```python
from build123d import *

# Parameters (mm, degrees)
BOSS_EXTRUDE1_DEPTH = 3.95
SKETCH2_R           = 3.575
CUT_EXTRUDE1_DEPTH  = 3.95
BOSS_EXTRUDE2_DEPTH = 1.64
SKETCH4_R           = 3.25
CUT_EXTRUDE2_DEPTH  = 63.643819328
CAVITY1_OUTLINE_R   = 3.25
CAVITY1_DEPTH       = 5.59
CAVITY1_START       = 3.19
CAVITY1_2_DEPTH     = 2.4
CUT_EXTRUDE4_DEPTH  = 63.643819328
BOSS_EXTRUDE3_START = -5.59
BOSS_EXTRUDE3_DEPTH = 5.59
BOSS_EXTRUDE4_DEPTH = 5.59
BOSS_EXTRUDE5_DEPTH = 5.59
CUT_EXTRUDE5_DEPTH  = 2.4
SKETCH7_R           = 1
CUT_EXTRUDE6_DEPTH  = 5.59


# Read off the part's stored shape, not the designer's step: Cavity1
with BuildPart() as part:
    # Sketch1 → Boss-Extrude1 (new body)
    with BuildSketch(Plane(origin=(0, 0, 0), x_dir=(1, 0, 0), z_dir=(0, 1, 0))):
        with BuildLine():
            Line((0, 7), (55, 7))
            ThreePointArc((55, 7), (62, 0), (55, -7))
            Line((55, -7), (0, -7))
            ThreePointArc((0, -7), (-7, 0), (0, 7))
        make_face()
    extrude(amount=BOSS_EXTRUDE1_DEPTH)

    # Sketch2 → Cut-Extrude1 (cut)
    with BuildSketch(Plane.XZ):
        with Locations(Location((0, 0, 0), (0, 0, 270))):
            Circle(SKETCH2_R)
    extrude(amount=-CUT_EXTRUDE1_DEPTH, mode=Mode.SUBTRACT)

    # Sketch3 → Boss-Extrude2 (add)
    with BuildSketch(Plane(origin=(0, 3.95, 0), x_dir=(1, 0, 0), z_dir=(0, 1, 0))):
        with BuildLine():
            Line((0, -7), (55, -7))
            ThreePointArc((55, -7), (62, 0), (55, 7))
            Line((55, 7), (0, 7))
            ThreePointArc((0, 7), (-7, 0), (0, -7))
        make_face()
        with BuildLine():
            Line((13.979308982, 2.569996388), (1.997926282, 3.167540934))
            ThreePointArc((1.997926282, 3.167540934), (-3.745, 0), (1.997926282, -3.167540934))
            Line((1.997926282, -3.167540934), (13.979308982, -2.569996388))
            ThreePointArc((13.979308982, -2.569996388), (16.545, 0), (13.979308982, 2.569996388))
        make_face(mode=Mode.SUBTRACT)
    extrude(amount=BOSS_EXTRUDE2_DEPTH)

    # Sketch4 → Cut-Extrude2 (cut, through all)
    with BuildSketch(Plane(origin=(0, 5.59, 0), x_dir=(1, 0, 0), z_dir=(0, 1, 0))):
        with Locations(Location((55, 0, 0), (0, 0, 270))):
            Circle(SKETCH4_R)
    extrude(amount=-CUT_EXTRUDE2_DEPTH, mode=Mode.SUBTRACT)

    # Cavity1 outline → Cavity1 (cut)
    with BuildSketch(Plane(origin=(0, 0, 0), x_dir=(1, 0, 0), z_dir=(0, 1, 0))):
        with BuildLine():
            Line((58.605551275, 6), (38, 6))
            Line((38, 6), (38, -6))
            Line((38, -6), (58.605551275, -6))
            ThreePointArc((58.605551275, -6), (59.949747468, -4.949747468), (61, -3.605551275))
            Line((61, -3.605551275), (61, 3.605551275))
            ThreePointArc((61, 3.605551275), (59.949747468, 4.949747468), (58.605551275, 6))
        make_face()
        with Locations((55, 0)):
            Circle(CAVITY1_OUTLINE_R, mode=Mode.SUBTRACT)
    extrude(amount=CAVITY1_DEPTH, mode=Mode.SUBTRACT)

    # Cavity1 2 outline → Cavity1 2 (cut)
    with BuildSketch(Plane(origin=(0, 0, 0), x_dir=(1, 0, 0), z_dir=(0, 1, 0)).offset(CAVITY1_START)):
        with BuildLine():
            Line((33.3, 0.5), (34.605619966, 0.5))
            ThreePointArc((34.605619966, 0.5), (36.47164537, 0), (34.605619966, -0.5))
            Line((34.605619966, -0.5), (33.3, -0.5))
            Line((33.3, -0.5), (33.3, -6))
            Line((33.3, -6), (38, -6))
            Line((38, -6), (38, 6))
            Line((38, 6), (33.3, 6))
            Line((33.3, 6), (33.3, 0.5))
        make_face()
        with BuildLine():
            ThreePointArc((61, -3.605551275), (62, 0), (61, 3.605551275))
            Line((61, 3.605551275), (61, -3.605551275))
        make_face()
    extrude(amount=CAVITY1_2_DEPTH, mode=Mode.SUBTRACT)

    # Sketch5 → Cut-Extrude4 (cut, through all)
    with BuildSketch(Plane.XZ):
        with BuildLine():
            Line((61, 3.605551275), (61, -3.605551275))
            ThreePointArc((61, -3.605551275), (62, 0), (61, 3.605551275))
        make_face()
    extrude(amount=-CUT_EXTRUDE4_DEPTH, mode=Mode.SUBTRACT)

    # Sketch6 → Boss-Extrude3 (add)
    with BuildSketch(Plane(origin=(0, 5.59, 0), x_dir=(1, 0, 0), z_dir=(0, 1, 0)).offset(BOSS_EXTRUDE3_START)):
        with BuildLine():
            Line((61, -6), (58.605551275, -6))
            ThreePointArc((58.605551275, -6), (56.870828693, -6.745368782), (55, -7))
            Line((55, -7), (66.7, -7))
            Line((66.7, -7), (66.7, 7))
            Line((66.7, 7), (55, 7))
            ThreePointArc((55, 7), (56.870828693, 6.745368782), (58.605551275, 6))
            Line((58.605551275, 6), (61, 6))
            Line((61, 6), (65.7, 6))
            Line((65.7, 6), (65.7, 0.5))
            Line((65.7, 0.5), (65.7, -0.5))
            Line((65.7, -0.5), (65.7, -6))
            Line((65.7, -6), (61, -6))
        make_face()
        with BuildLine():
            Line((58.605551275, -6), (33.3, -6))
            Line((33.3, -6), (33.3, -7))
            Line((33.3, -7), (55, -7))
            ThreePointArc((55, -7), (56.870828693, -6.745368782), (58.605551275, -6))
        make_face()
        with BuildLine():
            Line((33.3, 7), (33.3, 6))
            Line((33.3, 6), (58.605551275, 6))
            ThreePointArc((58.605551275, 6), (56.870828693, 6.745368782), (55, 7))
            Line((55, 7), (33.3, 7))
        make_face()
    extrude(amount=BOSS_EXTRUDE3_DEPTH)

    # Sketch6<3> → Boss-Extrude4 (add)
    with BuildSketch(Plane(origin=(0, 5.59, 0), x_dir=(1, 0, 0), z_dir=(0, 1, 0))):
        with BuildLine():
            Line((64.394380034, -0.5), (65.7, -0.5))
            Line((65.7, -0.5), (65.7, 0.5))
            Line((65.7, 0.5), (64.394380034, 0.5))
            ThreePointArc((64.394380034, 0.5), (62.52835463, 0), (64.394380034, -0.5))
        make_face()
    extrude(amount=-BOSS_EXTRUDE4_DEPTH)

    # Sketch6<5> → Boss-Extrude5 (add)
    with BuildSketch(Plane(origin=(0, 5.59, 0), x_dir=(1, 0, 0), z_dir=(0, 1, 0))):
        with BuildLine():
            Line((61, 6), (61, -6))
            Line((61, -6), (65.7, -6))
            Line((65.7, -6), (65.7, -0.5))
            Line((65.7, -0.5), (64.394380034, -0.5))
            ThreePointArc((64.394380034, -0.5), (62.52835463, 0), (64.394380034, 0.5))
            Line((64.394380034, 0.5), (65.7, 0.5))
            Line((65.7, 0.5), (65.7, 6))
            Line((65.7, 6), (61, 6))
        make_face()
    extrude(amount=-BOSS_EXTRUDE5_DEPTH)

    # Sketch6<6> → Cut-Extrude5 (cut)
    with BuildSketch(Plane(origin=(0, 5.59, 0), x_dir=(1, 0, 0), z_dir=(0, 1, 0))):
        with BuildLine():
            Line((61, 6), (61, -6))
            Line((61, -6), (65.7, -6))
            Line((65.7, -6), (65.7, -0.5))
            Line((65.7, -0.5), (64.394380034, -0.5))
            ThreePointArc((64.394380034, -0.5), (62.52835463, 0), (64.394380034, 0.5))
            Line((64.394380034, 0.5), (65.7, 0.5))
            Line((65.7, 0.5), (65.7, 6))
            Line((65.7, 6), (61, 6))
        make_face()
    extrude(amount=-CUT_EXTRUDE5_DEPTH, mode=Mode.SUBTRACT)

    # Sketch7 → Cut-Extrude6 (cut)
    with BuildSketch(Plane(origin=(0, 5.59, 0), x_dir=(1, 0, 0), z_dir=(0, 1, 0))):
        with Locations(Location((63.52835463, 0, 0), (0, 0, 270))):
            Circle(SKETCH7_R)
        with Locations(Location((35.47164537, 0, 0), (0, 0, 270))):
            Circle(SKETCH7_R)
    extrude(amount=-CUT_EXTRUDE6_DEPTH, mode=Mode.SUBTRACT)


solid = part.part
```
Geometry: final body of the model. Coordinates: model frame, mm. A direction names the side the tool comes from. Give positions to 0.01 mm unless a question says otherwise; leave off trailing zeros. Loops run counter-clockwise (first coordinate to the right, second up) from the corner with the lowest first, then second, coordinate; pieces in that order, holes last. Notation, with made-up numbers: (1.5, -21) -> (5.5, -21) arc R20 ccw to (5.5, 3) -> close; hole circle Ø10 at (20.25, -4.5). An arc over 180 degrees is marked (long way). Use CSV: the item, a comma, the result in double quotes.
(1) Cut plane C-C (y = 2.3). Output: boundary loops of the cut face in (x, z) (3 decimals).
From the geometry:
outline,"(0, -7) -> (66.7, -7) -> (66.7, 7) -> (0, 7) arc R7 ccw to start; hole circle Ø7.15 at (0, 0); hole circle Ø2 at (35.472, 0); hole (38, -6) -> (61, -6) -> (61, 6) -> (38, 6) -> close; hole circle Ø2 at (63.528, 0)"
(2) First-contact query: P1, Ø1.9, axis at y = 5, z = -3.5, coming from the -X side. Flat tip, straight axial feed; report the tip coordinate or a pass-through.
From the geometry:
P1,"x = -6.52"
(3) Pull-direction query (X, two-part tool) for faces 3 (the face through (-7, 3, 0)), 4 (the face through (34, 3, -7)), 5 (the face through (33.3, 4, -3)); classes: released by +X, released by -X, zero draft, split by the parting line, or undercut.
From the geometry:
face 3,"released by -X"
face 4,"zero draft"
face 5,"undercut"
(4) Access query for faces 1 (the face through (21, 5.59, 0)), 2 (the face through (16.544, 4.759, 0.056)). Directions: +Z, -Z, +X, -X, +Y, -Y. A direction counts if a zero-diameter tool reaches every point of the face in a straight line with its end or side. Return the directions, or none.
From the geometry:
face 1,"+Z, -Z, +X, -X, +Y"
face 2,"+Y"
(5) Ray query, line 1 along X through (y, z) = (1.55, 0) (3 decimals); line 2 along Z through (x, y) = (34, 4.45); line 3 along Z through (x, y) = (39.5, 2.8). Return the intervals inside material, ascending. Write a range as [from, to].
From the geometry:
line 1,"[-7, -3.575], [3.575, 34.472], [36.472, 38], [61, 62.528], [64.528, 66.7]"
line 2,"[-7, -6], [-0.5, 0.5], [6, 7]"
line 3,"[-7, -6], [6, 7]"
(6) Cut plane D-D (z = 1.75). Output: boundary loops of the cut face in (x, y).
From the geometry:
outline,"(-6.78, 0) -> (-3.12, 0) -> (-3.12, 3.95) -> (-3.31, 3.95) -> (-3.31, 5.59) -> (-6.78, 5.59) -> close; (3.12, 0) -> (38, 0) -> (38, 3.19) -> (33.3, 3.19) -> (33.3, 5.59) -> (15.86, 5.59) -> (15.86, 3.95) -> (3.12, 3.95) -> close; (61, 0) -> (66.7, 0) -> (66.7, 5.59) -> (65.7, 5.59) -> (65.7, 3.19) -> (61, 3.19) -> close"
(7) Cut plane A-A (x = 59). Output: boundary loops of the cut face in (y, z), plus the area to 3 significant figures.
From the geometry:
outline,"(0, -7) -> (5.59, -7) -> (5.59, -6) -> (0, -6) -> close; (0, 6) -> (5.59, 6) -> (5.59, 7) -> (0, 7) -> close"
area,"11.2 mm^2"
(8) Cut plane B-B (z = 4.5). Output: boundary loops of the cut face in (x, y).
From the geometry:
outline,"(-5.36, 0) -> (38, 0) -> (38, 3.19) -> (33.3, 3.19) -> (33.3, 5.59) -> (-5.36, 5.59) -> close; (61, 0) -> (66.7, 0) -> (66.7, 5.59) -> (65.7, 5.59) -> (65.7, 3.19) -> (61, 3.19) -> close"
